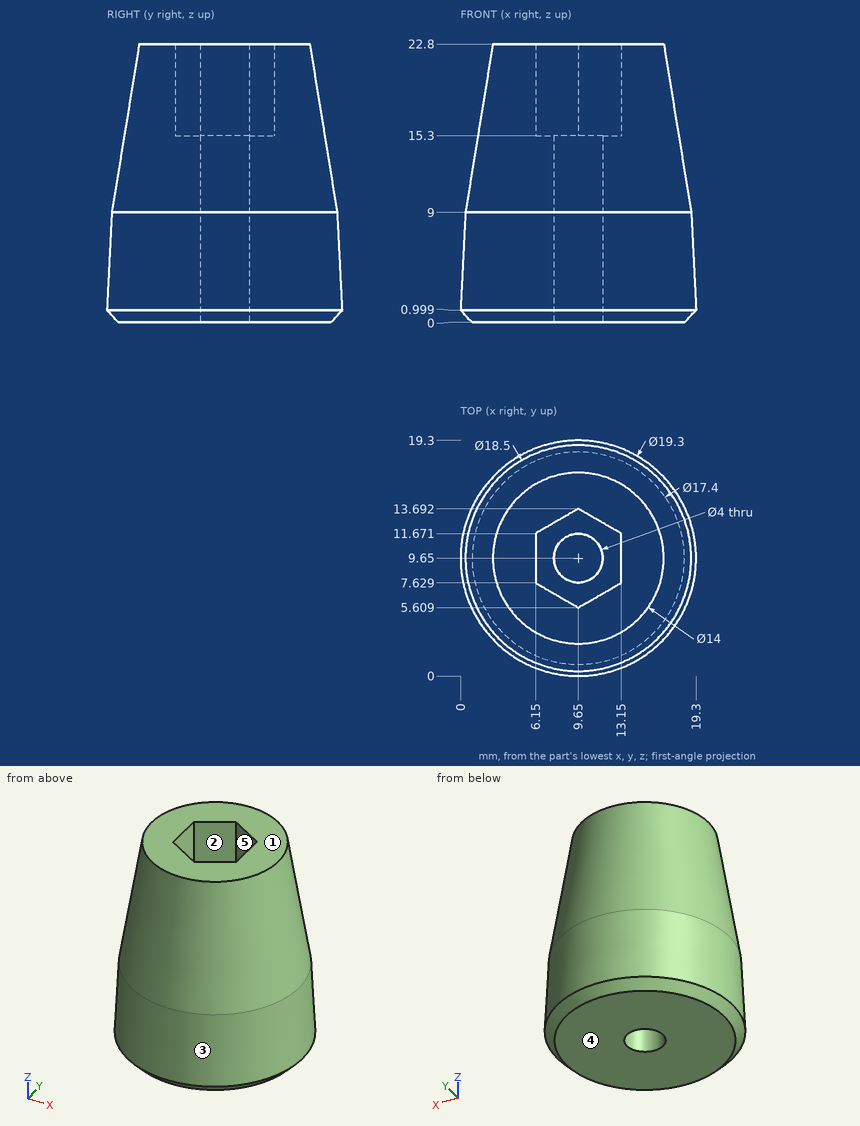
Can you work these out from the drawing? Everything is in mm from the part's minimum corner. A direction names the side the tool comes from. Coordinates: 2 decimals unless noted, no trailing zeros. Use a Markdown table: item, result.
Q1. I'm going to push flat-ended pins straight in: pin 1 Ø1 at (x, y) = (7, 11) entering from +Z; pin 2 Ø5 at (y, z) = (7.5, 10) entering from +X; pin 3 Ø3 at (y, z) = (10.5, 19) entering from -X; pin 4 Ø1.5 at (x, y) = (11.5, 7) entering from +Z. Where does each tip first touch, or does it pass through?
Geometry check:
| item | result |
|---|---|
| pin 1 | stops at z = 15.3 |
| pin 2 | stops at x = 18.93 |
| pin 3 | stops at x = 1.81 |
| pin 4 | stops at z = 22.8 |
Q2. Please list where these lines run through material, in increasing order: L1, parallel to Z at x = 9.75, y = 6.75; L2, parallel to Y at x = 10.25, z = 21.75 (1 decimal); L3, parallel to X at y = 8.5, z = 3.75 (1 decimal).
Geometry check:
| item | result |
|---|---|
| L1 | z = 0 to 15.3 |
| L2 | y = 2.5 to 6, 13.3 to 16.8 |
| L3 | x = 0.2 to 8, 11.3 to 19.1 |
Q3. Thinking about a two-plate mould opening in Y: for the marked faces 3, 4 and 5, which applies, +Y half, -Y half, draft (parallel to the pull), parting line (faces both ways), or undercut?
Geometry check:
| item | result |
|---|---|
| face 3 | parting line |
| face 4 | draft |
| face 5 | undercut |
Q4. Which directions (+Z, -Z, +X, -X, +Y, -Y) give clear straight access to the entire face, cutting with the end or side of a thin tool? Please do the marked faces 1 and 2.
Geometry check:
| item | result |
|---|---|
| face 1 | +Z, +X, -X, +Y, -Y |
| face 2 | +Z |
